Autodesk Inventor part; units mm, degrees
ref_plane "YZ Plane" through (0, 0, 0) normal (1, 0, 0) x (0, 1, 0)
ref_plane "XZ Plane" through (0, 0, 0) normal (0, 1, 0) x (-1, 0, 0)
ref_plane "XY Plane" through (0, 0, 0) normal (0, 0, 1) x (1, 0, 0)
sketch "Sketch1" plane through (0, 0, 0) normal (0, 1, 0) x (-1, 0, 0)
  line L0 (0, 0) -> (3.81, 0)
  line L1 (3.81, 0) -> (3.81, -50.8)
  line L2 (3.81, -50.8) -> (0, -50.8)
  line L3 (0, -50.8) -> (0, 0)
  line L4 (0, 0) -> (12.7, 0)
  line L5 (12.7, 0) -> (12.7, 8.89)
  line L6 (12.7, 8.89) -> (0, 8.89)
  line L7 (0, 8.89) -> (0, 0)
  line L8 (0, -50.8) -> (12.7, -50.8)
  line L9 (12.7, -50.8) -> (12.7, -59.69)
  line L10 (12.7, -59.69) -> (0, -59.69)
  line L11 (0, -59.69) -> (0, -50.8)
  dimension "d0" = 3.81
  dimension "d1" = 50.8
  dimension "d2" = 12.7
  dimension "d3" = 8.89
  dimension "d4" = 12.7
  dimension "d5" = 8.89
extrude "Extrusion1" add sketch "Sketch1" along normal blind 12.7
sketch "Sketch2" plane through (0, 0, 8.89) normal (1, 0, 0) x (0, 0, -1)
  line L0 (0, 12.7) -> (68.58, 12.7) construction
  line L1 (8.89, 0) -> (0, 0) construction
  line L2 (0, 0) -> (0, 12.7) construction
  line L3 (0, 12.7) -> (8.89, 12.7) construction
  line L4 (8.89, 12.7) -> (8.89, 0) construction
  line L5 (34.29, 12.7) -> (34.29, 0) construction
  line L6 (59.69, 0) -> (8.89, 0) construction
  point P0 (4.445, 6.35)
  point P1 (64.135, 6.35)
hole "Hole1" at (0, 6.35, 4.445) at (0, 6.35, -55.245) direction (-1, 0, 0) diameter 3.2766 end through all countersink diameter 5.715 countersink angle 82
fillet "Fillet1" radius 0.762 24 edges at (-6.35, 12.7, 8.89) (-6.35, 0, 8.89) (0, 6.35, 8.89) (0, 12.7, -25.4) (0, 0, -25.4) (0, 6.35, -59.69) (-8.255, 12.7, 0) (-3.81, 12.7, -25.4) (-8.255, 12.7, -50.8) (-12.7, 12.7, 4.445) (-12.7, 6.35, 8.89) (-6.35, 12.7, -59.69) (-6.35, 0, -59.69) (-8.255, 0, -50.8) (-8.255, 0, 0) (-3.81, 0, -25.4) (-12.7, 6.35, -50.8) (-12.7, 6.35, -59.69) (-12.7, 6.35, -53.6067) (-12.7, 12.7, -55.245) (-12.7, 0, -55.245) (-12.7, 0, 4.445) (-12.7, 6.35, 0) (-12.7, 6.35, 6.0833)
properties part number "PMSretainer"
Could you check a few things on this model? Use its own coordinates, in mm. A direction names the side the tool comes from. Give positions to 0.01 mm unless a question says otherwise; leave off trailing zeros. Order: outer loops, then holes, each group sorted by start corner. A loop starts at its lowest first (then second) coordinate and runs counter-clockwise, first axis right, second up.
1. For faces 5 (the flat face through (-8, 6, -50.8)), 6 (the flat face through (-12.7, 6, 7)), which set-ups out of +Z, -Z, +X, -X, +Y, -Y let a thin tool reach every point of the face, with its end or its side?
2. I need wall thicknesses on L1, parallel to Z at x = -7.75, y = 6.35; L2, parallel to Z at x = -4.75, y = 9.25; L3, parallel to Z at x = -3.5, y = 7.5. Which ranges of each line are inside material? Lowest first, please.
3. Suppose I cut it at D-D (z = -17). List the corners of the cut face in (x, y) for me.
4. Suppose I cut it at B-B (y = 6.35). Give the number of separate pieces and of enclosed holes in the cut face, plus the area to 3 significant figures.
5. We'd pull the mould along Z, two halves only. Please class faces 1 (the cylindrical face through (-6.74, 5.86, -56.81)), 2 (the flat face through (-6, 6, 8.89)), 3 (the flat face through (-12.7, 6, -58)), 4 (the flat face through (-8, 6, 0)): pulls with the +Z half, pulls with the -Z half, needs draft (parallel to the pull), parting line crosses it, or undercut.
6. Will these pins go through, and if not, where does the flat tip stop? P1, Ø3, axis at y = 9.5, z = -46.5, coming from the -X side; P2, Ø6, axis at y = 5, z = -36, coming from the +X side; P3, Ø5, axis at y = 6.35, z = 4.445, coming from the +X side.
7. Suppose I cut it at A-A (x = -9.25). List the corners of the cut face in (y, z) for me (3 decimals).
8. Suppose I cut it at C-C (x = -2). List the corners of the cut face in (y, z) for me (3 decimals).
Solved:
1. face 5: -X, +Y, -Y
1. face 6: +Z, -Z, -X, +Y, -Y
2. L1: z = -59.69 to -56.88, -53.61 to -50.8, 0 to 2.81, 6.08 to 8.89
2. L2: z = -59.69 to -50.8, 0 to 8.89
2. L3: z = -59.69 to -56.41, -54.08 to 3.28, 5.61 to 8.89
3. outline: (-3.81, 0.76) arc R0.76 ccw to (-3.05, 0) - (-0.76, 0) arc R0.76 ccw to (0, 0.76) - (0, 11.94) arc R0.76 ccw to (-0.76, 12.7) - (-3.05, 12.7) arc R0.76 ccw to (-3.81, 11.94) - close
4. separate pieces: 3
4. enclosed holes: 0
4. area: 331 mm2
5. face 1: undercut
5. face 2: pulls with the +Z half
5. face 3: needs draft
5. face 4: undercut
6. P1: stops at x = -3.81
6. P2: stops at x = 0
6. P3: stops at x = -0.41
7. outline: (0, -58.928) arc R0.762 ccw to (0.762, -59.69) - (11.938, -59.69) arc R0.762 ccw to (12.7, -58.928) - (12.7, -51.562) arc R0.762 ccw to (11.938, -50.8) - (0.762, -50.8) arc R0.762 ccw to (0, -51.562) - close; (0, 0.762) arc R0.762 ccw to (0.762, 0) - (11.938, 0) arc R0.762 ccw to (12.7, 0.762) - (12.7, 8.128) arc R0.762 ccw to (11.938, 8.89) - (0.762, 8.89) arc R0.762 ccw to (0, 8.128) - close; hole circle Ø3.277 at (6.35, -55.245); hole circle Ø3.277 at (6.35, 4.445)
8. outline: (0, -58.928) arc R0.762 ccw to (0.762, -59.69) - (11.938, -59.69) arc R0.762 ccw to (12.7, -58.928) - (12.7, 8.128) arc R0.762 ccw to (11.938, 8.89) - (0.762, 8.89) arc R0.762 ccw to (0, 8.128) - close; hole circle Ø3.277 at (6.35, -55.245); hole circle Ø3.277 at (6.35, 4.445)
